Read the model definition and answer for the solid it produces. Units are mm, in the model's axes. Face numbers are marked on the shaded views. A direction names the side the tool comes from. Give positions to 0.01 mm unless a question says otherwise; leave off trailing zeros. Loops run counter-clockwise (first coordinate to the right, second up) from the corner with the lowest first, then second, coordinate; pieces in that order, holes last. Notation, with made-up numbers: (-9, -40) -> (-4, -40) arc R24 ccw to (-4, -10) -> close; hole circle Ø4 at (53, 45.25). An arc over 180 degrees is marked (long way). Write each question's results on one line, items separated by ' | '. Start each with the question number.
Item 1: Determine the mould class of the marked faces 4, 5 and 6 for opening direction X: +X half, -X half, draft (parallel to the pull), parting line (faces both ways), or undercut.
Item 2: Section D-D on x = 0 is taken. Write down the section's boundary in (y, z).
Item 3: Section A-A on x = 23 is taken. Write down the section's boundary in (y, z), and give its area (3 significant figures).
Item 4: Each of these flat-tipped pins is pushed along its axis until it touches: P1, Ø1.5, axis at y = 12, z = 2, coming from the -X side; P2, Ø1.8, axis at x = -24, z = 3.5, coming from the +Y side; P3, Ø1, axis at y = 5, z = 1, coming from the -X side. Where does it stop, or does it pass through?
Item 5: Section C-C on y = 4.5 is taken. Write down the section's boundary in (x, z), and give its area (3 significant figures).
Item 6: Find the intervals of material crossed by line 1 (Z direction, x = 23, y = 0.6); line 2 (X direction, y = 4.5, z = 2.2); line 3 (Y direction, x = 20.5, z = 4.45), in increasing order.
Item 7: Which of the six approach directions +Z, -Z, +X, -X, +Y, -Y give full straight-line access (tool end or side, diameter ignored) to the marked faces 1, 2 and 3?
Item 8: Section B-B on z = 3 is taken. Write down the section's boundary in (x, y), and give its area (3 significant figures).
```python
from build123d import *

# Parameters (mm, degrees)
PAD_DEPTH   = 6
SKETCH001_R = 1.65
HOLE_DEPTH  = 25


with BuildPart() as part:
    # Sketch → Pad (new body)
    with BuildSketch(Plane.XY):
        with BuildLine():
            ThreePointArc((10.5, 0), (0, 10.5), (-10.5, 0))
            Line((-27.5, 0), (-10.5, 0))
            Line((-27.5, 3), (-27.5, 0))
            Line((-18.761663, 3), (-27.5, 3))
            ThreePointArc((18.761663, 3), (0, 19), (-18.761663, 3))
            Line((27.5, 3), (18.761663, 3))
            Line((27.5, 0), (27.5, 3))
            Line((27.5, 0), (10.5, 0))
        make_face()
    extrude(amount=PAD_DEPTH)

    # Sketch001 (on Face5 of Pad) → Hole (cut)
    with BuildSketch(Plane(origin=(0, 3, 0), x_dir=(-1, 0, 0), z_dir=(0, 1, 0))):
        with Locations((-23, 3)):
            Circle(SKETCH001_R)
        with Locations((23, 3)):
            Circle(SKETCH001_R)
    extrude(amount=-HOLE_DEPTH, mode=Mode.SUBTRACT)


solid = part.part
```
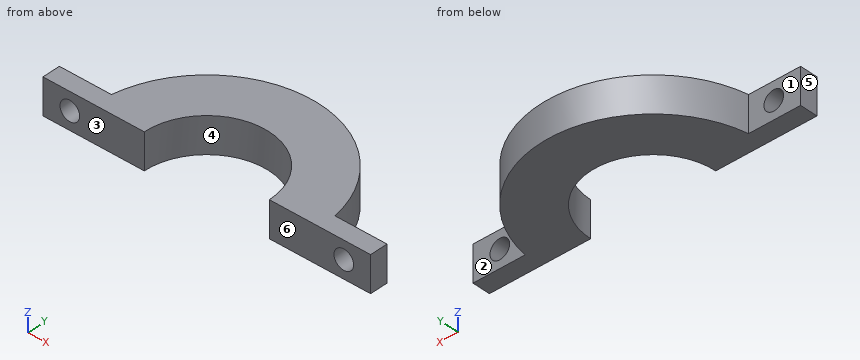
Findings:
1) face 4: undercut | face 5: -X half | face 6: draft
2) outline: (10.5, 0) -> (19, 0) -> (19, 6) -> (10.5, 6) -> close
3) outline: (0, 0) -> (3, 0) -> (3, 1.35) -> (0, 1.35) -> close; (0, 4.65) -> (3, 4.65) -> (3, 6) -> (0, 6) -> close | area: 8.10 mm2
4) P1: x = -15.31 | P2: y = 3 | P3: x = -18.46
5) outline: (-18.46, 0) -> (-9.49, 0) -> (-9.49, 6) -> (-18.46, 6) -> close; (9.49, 0) -> (18.46, 0) -> (18.46, 6) -> (9.49, 6) -> close | area: 108 mm2
6) line 1: 0 to 1.35, 4.65 to 6 | line 2: -18.46 to -9.49, 9.49 to 18.46 | line 3: 0 to 3
7) face 1: +Z, -Z, -X, +Y | face 2: +Z, -Z, +X, +Y | face 3: +Z, -Z, +X, -X, -Y
8) outline: (-27.5, 0) -> (-24.65, 0) -> (-24.65, 3) -> (-27.5, 3) -> close; (-21.35, 0) -> (-10.5, 0) arc R10.5 cw to (10.5, 0) -> (21.35, 0) -> (21.35, 3) -> (18.76, 3) arc R19 ccw to (-18.76, 3) -> (-21.35, 3) -> close; (24.65, 0) -> (27.5, 0) -> (27.5, 3) -> (24.65, 3) -> close | area: 426 mm2
